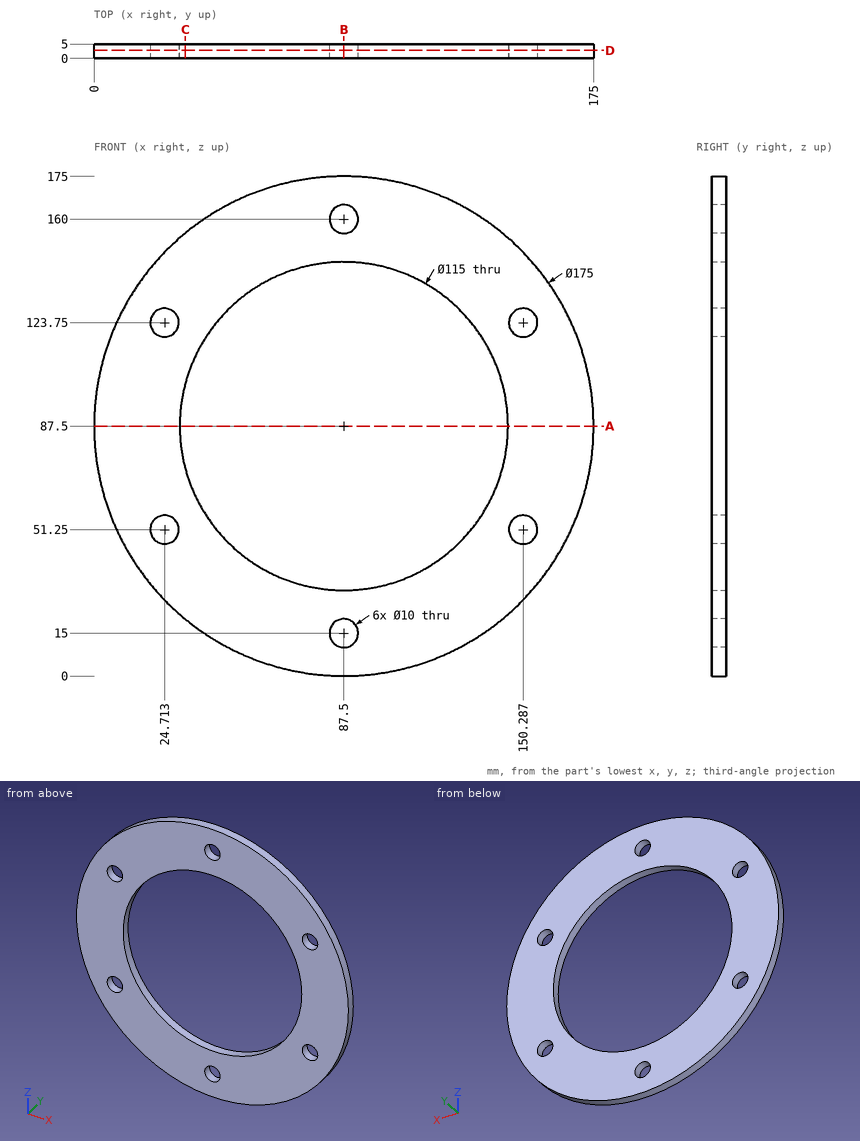
The drawing under review shows one solid part. Ordinate dimensions are in mm from its lowest x, y, z. Round coordinates to 2 decimals unless told otherwise and drop trailing zeros. Loops run counter-clockwise (first coordinate to the right, second up) from the corner with the lowest first, then second, coordinate; pieces in that order, holes last. Notation, with made-up numbers: (30, 58) - (84, 58) arc R29 ccw to (84, 90) - close; hole circle Ø11 at (61, 24.5). An arc over 180 degrees is marked (long way). Put each result on its own line as item: value. Start each with the question number.
1. Consider section D-D on y = 2.75. State the section outline as (x, z) points.
2. Consider section C-C on x = 32. State the section outline as (y, z) points.
3. For probe 1 along X at (y, z) = (1.35, 86); probe 2 along Z at (x, y) = (24, 3.95); probe 3 along Z at (x, y) = (25, 4.2), list the stretches that pass through material, from the lowest coordinate up. Write a range as [from, to].
4. Consider section A-A on z = 87.5. State the section outline as (x, y) points.
5. Consider section B-B on x = 87.5. State the section outline as (y, z) points.
6. Insertion check: P1, Ø3, axis at x = 52, y = 2.5, coming from the -Z side; P2, Ø13, axis at x = 87.5, z = 15, coming from the +Y side; P3, Ø3, axis at y = 3.5, z = 28, coming from the +X side (1 decimal); P4, Ø6, axis at x = 24.71, z = 123.75, coming from the +Y side. Each pin has a flat end and moves straight along its axis. Give the tip position at first contact, or say it passes through.
Result sheet:
1. outline: circle Ø175 at (87.5, 87.5); hole circle Ø10 at (24.71, 51.25); hole circle Ø10 at (24.71, 123.75); hole circle Ø115 at (87.5, 87.5); hole circle Ø10 at (87.5, 15); hole circle Ø10 at (87.5, 160); hole circle Ø10 at (150.29, 51.25); hole circle Ø10 at (150.29, 123.75)
2. outline: (0, 19.85) - (5, 19.85) - (5, 72.47) - (0, 72.47) - close; (0, 102.53) - (5, 102.53) - (5, 155.15) - (0, 155.15) - close
3. probe 1: [0.01, 30.02], [144.98, 174.99]
3. probe 2: [27.3, 46.3], [56.2, 118.8], [128.7, 147.7]
3. probe 3: [26.26, 46.26], [56.24, 118.76], [128.74, 148.74]
4. outline: (0, 0) - (30, 0) - (30, 5) - (0, 5) - close; (145, 0) - (175, 0) - (175, 5) - (145, 5) - close
5. outline: (0, 0) - (5, 0) - (5, 10) - (0, 10) - close; (0, 20) - (5, 20) - (5, 30) - (0, 30) - close; (0, 145) - (5, 145) - (5, 155) - (0, 155) - close; (0, 165) - (5, 165) - (5, 175) - (0, 175) - close
6. P1: z = 6.88
6. P2: y = 5
6. P3: x = 153
6. P4: through
